Can you work these out from the drawing? Everything is in mm from the part's minimum corner. A direction names the side the tool comes from. Give positions to 0.01 mm unless a question says otherwise; leave off trailing zeros. Write each loop counter-clockwise with the first axis right and the second up, starting at its lowest first coordinate (ties: lowest second). Pieces come first, ordered by that corner, then holes. Notation, with made-up numbers: (38, 6.5) -> (93, 6.5) arc R25 cw to (93, 40.5) -> close; hole circle Ø4 at (17.5, 85). An arc over 180 degrees is marked (long way). Return JSON: item names as keys, results as strings.
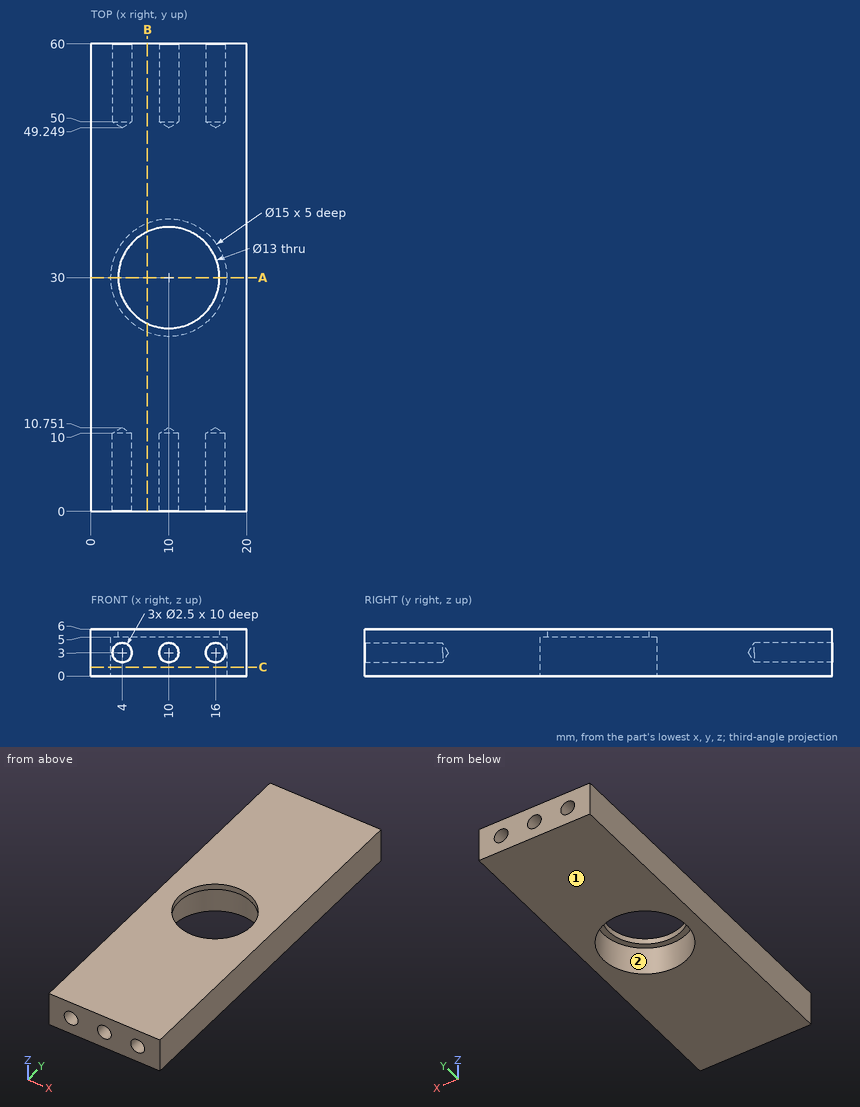
1. For pin 1 Ø1.5 at (x, z) = (16, 3) entering from -Y; pin 2 Ø2 at (x, y) = (4, 32) entering from -Z; pin 3 Ø1.5 at (x, z) = (4, 3) entering from +Y, each with a flat end and sliding along its axis, tell me the tip position at first contact or that it passes through.
Taken from the geometry:
{"pin 1": "stops at y = 10.3", "pin 2": "stops at z = 5", "pin 3": "stops at y = 49.7"}
2. Suppose I cut it at B-B, the plane x = 7.25. List the corners of the cut face in (y, z) for me.
Taken from the geometry:
{"outline": "(0, 0) -> (23.02, 0) -> (23.02, 5) -> (24.11, 5) -> (24.11, 6) -> (0, 6) -> close; (35.89, 5) -> (36.98, 5) -> (36.98, 0) -> (60, 0) -> (60, 6) -> (35.89, 6) -> close"}
3. Suppose I cut it at A-A, the plane y = 30. List the corners of the cut face in (x, z) for me.
Taken from the geometry:
{"outline": "(0, 0) -> (2.5, 0) -> (2.5, 5) -> (3.5, 5) -> (3.5, 6) -> (0, 6) -> close; (16.5, 5) -> (17.5, 5) -> (17.5, 0) -> (20, 0) -> (20, 6) -> (16.5, 6) -> close"}
4. Which directions (+Z, -Z, +X, -X, +Y, -Y) give clear straight access to the entire face, cutting with the end or side of a thin tool? Please do the marked faces 1 and 2.
Taken from the geometry:
{"face 1": "-Z, +X, -X, +Y, -Y", "face 2": "-Z"}
5. If I drill on line 1 (Y direction, x = 10, z = 5.65); line 2 (Z direction, x = 16, y = 4.5); line 3 (Y direction, x = 7.25, z = 2.95), over which ranges is the centre line in solid material (lowest first)? Write a range as [from, to].
Taken from the geometry:
{"line 1": "y = [0, 23.5], [36.5, 60]", "line 2": "z = [0, 1.75], [4.25, 6]", "line 3": "y = [0, 23.02], [36.98, 60]"}
6. Suppose I cut it at C-C, the plane z = 1.15. List the corners of the cut face in (x, y) for me.
Taken from the geometry:
{"outline": "(0, 0) -> (20, 0) -> (20, 60) -> (0, 60) -> close; hole circle Ø15 at (10, 30)"}
